Verification items for the finished model (mm, model axes). A direction names the side the tool comes from. Give positions to 0.01 mm unless a question says otherwise; leave off trailing zeros. Loops run counter-clockwise (first coordinate to the right, second up) from the corner with the lowest first, then second, coordinate; pieces in that order, holes last. Notation, with made-up numbers: (-21.75, -28) - (9.25, -28) arc R22 ccw to (9.25, -15) - close; hole circle Ø11 at (-35, 59). An arc over 180 degrees is marked (long way). One line per item, written item: value. Start each with the question number.
1. Sectioned sample at C-C (y = 35). Record the cut outline in (x, z) (3 decimals), plus the area to 3 significant figures.
2. Gauge pin test, flat ends, axial feed: pin 1 (5.5 mm diameter, centred on x = 0, z = -8.15, fed in from +Y); pin 2 (2.5 mm diameter, centred on x = 6.72, z = 6.72, fed in from +Y); pin 3 (2 mm diameter, centred on x = 0, z = -0.5, fed in from -Y). Record the tip position at first contact, or that the pin passes through.
3. Scan lines: L1, parallel to X at y = 22.85, z = 0; L2, parallel to Y at x = -3.25, z = 6; L3, parallel to Y at x = -7.75, z = 2.5. Record each from-to range of solid material in increasing order. Write a range as [from, to].
4. Access from +Z, -Z, +X, -X, +Y, -Y to the whole of each face (thin tool, end or side, straight path). Record for faces 1 (the flat face through (-11, 2.6, 0)), 2 (the flat face through (0, 2.6, 11)), 3 (the cylindrical face through (-2.89, 25.99, -3.77)).
5. Mould release check, pull along Z, two halves, no side actions. Record for faces 4 (the cylindrical face through (-0.1, 1.3, 8.4)), 5 (the flat face through (0, 1, 0)), 6 (the flat face through (3, 0, -5)), 7 (the flat face through (-7, 1, -7)): pulls with the +Z half, pulls with the -Z half, needs draft (parallel to the pull), parting line crosses it, or undercut.
6. Sectioned sample at D-D (y = 4). Record the cut outline in (x, z).
from build123d import *

# Parameters (mm, degrees)
SKETCH1_R           = 14
BOSS_EXTRUDE1_DEPTH = 25
CHAMFER1_SIZE       = 3.5
CHAMFER1_SIZE2      = 6.062177826
SKETCH2_R           = 4.75
BOSS_EXTRUDE2_DEPTH = 2
SKETCH3_R           = 1.575
BOSS_EXTRUDE3_DEPTH = 12
SKETCH4_R           = 11
CUT_EXTRUDE1_DEPTH  = 2.6
SKETCH5_R           = 1.5
SKETCH5_R_2         = 3.5
CUT_EXTRUDE2_DEPTH  = 1
CHAMFER2_SIZE       = 2
CHAMFER2_SIZE2      = 0.975465177
FILLET1_R           = 0.2
SKETCH6_R           = 3.15
CUT_EXTRUDE3_DEPTH  = 3


with BuildPart() as part:
    # Sketch1 → Boss-Extrude1 (new body)
    with BuildSketch(Plane(origin=(0, 0, 0), x_dir=(1, 0, 0), z_dir=(0, 1, 0))):
        with Locations(Location((0, 0, 0), (0, 0, 270))):
            Circle(SKETCH1_R)
    extrude(amount=BOSS_EXTRUDE1_DEPTH)

    # Chamfer1
    chamfer1_edges = [part.edges().sort_by_distance(p)[0] for p in [
        (0, 25, -14),
    ]]
    chamfer1_side = [part.faces().sort_by_distance(p)[0] for p in [
        (0, 12.5, -14),
    ]]
    chamfer(chamfer1_edges, length=CHAMFER1_SIZE, length2=CHAMFER1_SIZE2, reference=chamfer1_side[0])

    # Sketch2 → Boss-Extrude2 (add)
    with BuildSketch(Plane(origin=(0, 25, 0), x_dir=(1, 0, 0), z_dir=(0, 1, 0))):
        with Locations(Location((0, 0, 0), (0, 0, 270))):
            Circle(SKETCH2_R)
    extrude(amount=BOSS_EXTRUDE2_DEPTH)

    # Sketch3 → Boss-Extrude3 (add)
    with BuildSketch(Plane(origin=(0, 27, 0), x_dir=(1, 0, 0), z_dir=(0, 1, 0))):
        with Locations(Location((0, 0, 0), (0, 0, 270))):
            Circle(SKETCH3_R)
    extrude(amount=BOSS_EXTRUDE3_DEPTH)

    # Sketch4 → Cut-Extrude1 (cut)
    with BuildSketch(Plane.XZ):
        with Locations((-19.4, 0)):
            Circle(SKETCH4_R)
        with Locations((0, 19.4)):
            Circle(SKETCH4_R)
        with Locations((19.4, 0)):
            Circle(SKETCH4_R)
        with Locations((0, -19.4)):
            Circle(SKETCH4_R)
    extrude(amount=-CUT_EXTRUDE1_DEPTH, mode=Mode.SUBTRACT)

    # Sketch5 → Cut-Extrude2 (cut)
    with BuildSketch(Plane.XZ):
        with Locations(Location((-6.717514421, -6.717514421, 0), (0, 0, 270))):
            Circle(SKETCH5_R)
        with Locations(Location((-5.656854249, 5.656854249, 0), (0, 0, 270))):
            Circle(SKETCH5_R)
        with Locations(Location((6.717514421, 6.717514421, 0), (0, 0, 270))):
            Circle(SKETCH5_R)
        with Locations(Location((5.656854249, -5.656854249, 0), (0, 0, 270))):
            Circle(SKETCH5_R)
        with Locations(Location((0, 0, 0), (0, 0, 270))):
            Circle(SKETCH5_R_2)
    extrude(amount=-CUT_EXTRUDE2_DEPTH, mode=Mode.SUBTRACT)

    # Chamfer2
    chamfer2_edges = [part.edges().sort_by_distance(p)[0] for p in [
        (0, 0, 3.5),
    ]]
    chamfer2_side = [part.faces().sort_by_distance(p)[0] for p in [
        (0, 0, 8.070969364),
    ]]
    chamfer(chamfer2_edges, length=CHAMFER2_SIZE, length2=CHAMFER2_SIZE2, reference=chamfer2_side[0])

    # Fillet1
    fillet1_edges = [part.edges().sort_by_distance(p)[0] for p in [
        (0, 39, -1.575),
    ]]
    fillet(fillet1_edges, radius=FILLET1_R)

    # Sketch6 → Cut-Extrude3 (cut)
    with BuildSketch(Plane(origin=(0, 25, 0), x_dir=(1, 0, 0), z_dir=(0, 1, 0))):
        with Locations(Location((-8.15, 0, 0), (0, 0, 270))):
            Circle(SKETCH6_R)
        with Locations(Location((0, 8.15, 0), (0, 0, 270))):
            Circle(SKETCH6_R)
        with Locations(Location((8.15, 0, 0), (0, 0, 270))):
            Circle(SKETCH6_R)
        with Locations(Location((0, -8.15, 0), (0, 0, 270))):
            Circle(SKETCH6_R)
    extrude(amount=-CUT_EXTRUDE3_DEPTH, mode=Mode.SUBTRACT)


solid = part.part
Results are:
1. outline: circle Ø3.15 at (0, 0)
1. area: 7.79 mm^2
2. pin 1: stops at y = 22
2. pin 2: stops at y = 24.82
2. pin 3: stops at y = 1
3. L1: x = [-11.66, -11.3], [-5, 5], [11.3, 11.66]
3. L2: y = [0, 25]
3. L3: y = [0, 22]
4. face 1: -X, -Y
4. face 2: +Z, -Y
4. face 3: +Y
5. face 4: pulls with the +Z half
5. face 5: undercut
5. face 6: needs draft
5. face 7: undercut
6. outline: circle Ø28 at (0, 0)
